Build history of the part. All positions in model axes, mm. Face numbers are marked on the shaded views. A direction names the side the tool comes from. Give positions to 0.01 mm unless a question says otherwise; leave off trailing zeros. Order: outer loops, then holes, each group sorted by start corner. A loop starts at its lowest first (then second) coordinate and runs counter-clockwise, first axis right, second up. Notation, with made-up numbers: (24.5, 35) -> (80.5, 35) arc R11 cw to (80.5, 43) -> close; hole circle Ø4 at (17.5, 81.25). An arc over 180 degrees is marked (long way). One line per item, written item: value. Start each with the question number.
(1) Saw through at D-D on z = 0.25. Give the cut face in (x, y).
(2) Probe line 1 (Z direction, x = 4.75, y = 6); line 2 (X direction, y = 1.5, z = 4.25); line 3 (Y direction, x = 5.75, z = 2.25). List the from-to ranges inside material, lowest first.
(3) Two-plate mould, pull along X, no slides. Class the marked faces 1, 2, 3 and 4: +X half, -X half, draft (parallel to the pull), parting line (faces both ways), or undercut.
(4) Pin check, flat tips, straight feed: pin 1 (4 mm diameter, centred on y = 3.59, z = 5.12, fed in from -X); pin 2 (4 mm diameter, centred on x = 3, z = 4, fed in from -Y). Stop position of each tip, or through.
(5) Which spindle directions (+Z, -Z, +X, -X, +Y, -Y) get a long thin tool onto all of the face, cutting with end or side? Do the marked faces 5 and 6. Say none if no direction does.
(6) Saw through at B-B on x = 3. Give the cut face in (y, z).
(7) Saw through at A-A on y = 6.5. Give the cut face in (x, z), plus the area to 3 significant figures.
(8) Saw through at C-C on z = 3.5. Give the cut face in (x, y).
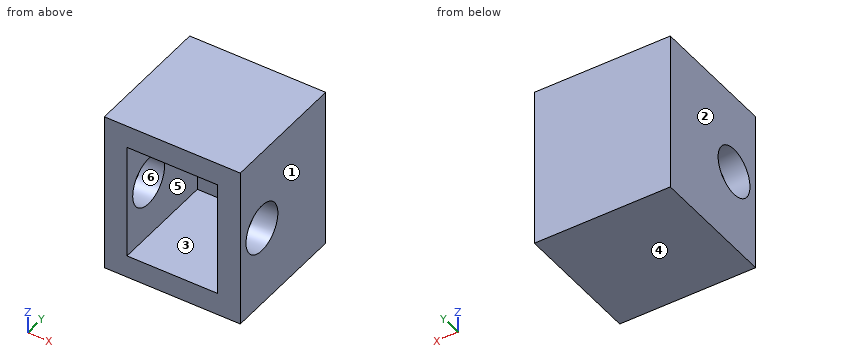
```python
from build123d import *

# Parameters (mm, degrees)
BOSS_EXTRUDE1_DEPTH = 10.24636
SKETCH2_R           = 2.12471
CUT_EXTRUDE1_DEPTH  = 12.99896
SKETCH3_W           = 10.24636
SKETCH3_H           = 0.6985
CUT_EXTRUDE2_DEPTH  = 12.99896
SKETCH4_W           = 1.99898
SKETCH4_H           = 11.38936
BOSS_EXTRUDE2_DEPTH = 11.99896


with BuildPart() as part:
    # Sketch1 → Boss-Extrude1 (new body)
    with BuildSketch(Plane.XY):
        Polygon((0, 0), (0, 10.08888), (8.001, 10.08888), (8.001, 0), (9.99998, 0), (9.99998, 12.08786), (-1.99898, 12.08786), (-1.99898, 0), align=None)
    extrude(amount=BOSS_EXTRUDE1_DEPTH)

    # Sketch2 → Cut-Extrude1 (cut, through all)
    with BuildSketch(Plane(origin=(9.99998, 0, 0), x_dir=(0, 0, -1), z_dir=(1, 0, 0))):
        with Locations((-5.12318, 3.58648)):
            Circle(SKETCH2_R)
    extrude(amount=-CUT_EXTRUDE1_DEPTH, mode=Mode.SUBTRACT)

    # Sketch3 → Cut-Extrude2 (cut, through all)
    with BuildSketch(Plane(origin=(9.99998, 0, 0), x_dir=(0, 0, -1), z_dir=(1, 0, 0))):
        with Locations((-5.12318, 0.34925)):
            Rectangle(SKETCH3_W, SKETCH3_H)
    extrude(amount=-CUT_EXTRUDE2_DEPTH, mode=Mode.SUBTRACT)

    # Sketch4 → Boss-Extrude2 (add)
    with BuildSketch(Plane(origin=(9.99998, 0, 0), x_dir=(0, 0, -1), z_dir=(1, 0, 0))):
        with Locations((-11.24585, 6.39318)):
            Rectangle(SKETCH4_W, SKETCH4_H)
        with Locations((0.99949, 6.39318)):
            Rectangle(SKETCH4_W, SKETCH4_H)
    extrude(amount=-BOSS_EXTRUDE2_DEPTH)


solid = part.part
```
Results below:
1. outline: (-2, 0.7) -> (0, 0.7) -> (0, 10.09) -> (8, 10.09) -> (8, 0.7) -> (10, 0.7) -> (10, 12.09) -> (-2, 12.09) -> close
2. line 1: z = -2 to 0, 10.25 to 12.25
2. line 2: x = -2 to 0, 8 to 10
2. line 3: y = 10.09 to 12.09
3. face 1: +X half
3. face 2: -X half
3. face 3: undercut
3. face 4: draft
4. pin 1: passes through
4. pin 2: stops at y = 10.09
5. face 5: -Y
5. face 6: +X, -X
6. outline: (0.7, -2) -> (12.09, -2) -> (12.09, 12.25) -> (0.7, 12.25) -> (0.7, 10.25) -> (10.09, 10.25) -> (10.09, 0) -> (0.7, 0) -> close
7. outline: (-2, -2) -> (10, -2) -> (10, 12.25) -> (-2, 12.25) -> close; hole (0, 0) -> (8, 0) -> (8, 10.25) -> (0, 10.25) -> close
7. area: 88.9 mm²
8. outline: (-2, 0.7) -> (0, 0.7) -> (0, 2.22) -> (-2, 2.22) -> close; (-2, 4.96) -> (0, 4.96) -> (0, 10.09) -> (8, 10.09) -> (8, 4.96) -> (10, 4.96) -> (10, 12.09) -> (-2, 12.09) -> close; (8, 0.7) -> (10, 0.7) -> (10, 2.22) -> (8, 2.22) -> close
